from build123d import *

# Parameters (mm, degrees)
F0_R     = 4.699
F1_DEPTH = 19.05
F2_DEPTH = 50.8
F3_DEPTH = 25.4


# Not quite as in the source:
# - a feature of the source that left no trace in its solid (it failed there, or was rolled back) is left out


with BuildPart() as f1:
    # F0 (on Top) → F1 (new body)
    with BuildSketch(Plane.XY):
        Polygon((46.0592823896, 54.4316620976), (-30.1407176104, 54.4316620976), (-30.1407176104, 29.0316620976), (-6.3155176104, 29.0316620976), (22.2340823896, 29.0316620976), (46.0592823896, 29.0316620976), align=None)
        with Locations((-17.4028014716, 41.883985333)):
            Circle(F0_R, mode=Mode.SUBTRACT)
        with Locations((33.3109036978, 41.7761531395)):
            Circle(F0_R, mode=Mode.SUBTRACT)
        Polygon((-6.3155176104, 29.0316620976), (-30.1407176104, 29.0316620976), (-30.1407176104, 3.6316620976), (-6.3155176104, 3.6316620976), (-6.3155176104, 16.6544260591), align=None)
        Polygon((-6.3155176104, 3.6316620976), (-30.1407176104, 3.6316620976), (-30.1407176104, -27.9789566994), (-30.1407176104, -40.8183379024), (-23.7907176104, -40.8183379024), (-17.4407176104, -40.8183379024), (33.3592823896, -40.8183379024), (46.0592823896, -40.8183379024), (46.0592823896, -28.1183379024), (46.0592823896, 3.6316620976), (22.2340823896, 3.6316620976), align=None)
        with Locations((-17.4763201279, -28.1499404974)):
            Circle(F0_R, mode=Mode.SUBTRACT)
        with Locations((33.0586231201, -27.9913925288)):
            Circle(F0_R, mode=Mode.SUBTRACT)
        Polygon((46.0592823896, 3.6316620976), (46.0592823896, 29.0316620976), (22.2340823896, 29.0316620976), (22.2340823896, 18.1238111109), (22.2340823896, 3.6316620976), align=None)
    extrude(amount=F1_DEPTH)

    # F0 (on Top) → F2 (join)
    with BuildSketch(Plane.XY):
        Polygon((-6.3155176104, 29.0316620976), (-30.1407176104, 29.0316620976), (-30.1407176104, 3.6316620976), (-6.3155176104, 3.6316620976), (-6.3155176104, 16.6544260591), align=None)
        Polygon((46.0592823896, 3.6316620976), (46.0592823896, 29.0316620976), (22.2340823896, 29.0316620976), (22.2340823896, 18.1238111109), (22.2340823896, 3.6316620976), align=None)
    extrude(amount=F2_DEPTH)

    # F0 (on Top) → F3 (join)
    with BuildSketch(Plane.XY):
        Polygon((22.2340823896, 29.0316620976), (-6.3155176104, 29.0316620976), (-6.3155176104, 16.6544260591), (-6.3155176104, 3.6316620976), (22.2340823896, 3.6316620976), (22.2340823896, 18.1238111109), align=None)
    extrude(amount=F3_DEPTH)


solid = f1.part
For this review, take the finished solid that the model builds, in its own axes (mm). A direction names the side the tool comes from. Round coordinates to 2 decimals unless told otherwise and drop trailing zeros. Loops run counter-clockwise (first coordinate to the right, second up) from the corner with the lowest first, then second, coordinate; pieces in that order, holes last. Notation, with made-up numbers: (43, 18) - (96, 18) arc R14 cw to (96, 37) - close; hole circle Ø1 at (11.25, -15). An arc over 180 degrees is marked (long way). Use one line per item in the form item = value.
1) We need section B-B on y = 23.5. Write out the cut boundary in (x, z), then the cut area to 3 significant figures.
Solutions:
outline = (-30.14, 0) - (46.06, 0) - (46.06, 50.8) - (22.23, 50.8) - (22.23, 25.4) - (-6.32, 25.4) - (-6.32, 50.8) - (-30.14, 50.8) - close
area = 3,150 mm2
2) We need section A-A on z = 32.5. Write out the cut boundary in (x, y), then the cut area to 3 significant figures.
Solutions:
outline = (-30.14, 3.63) - (-6.32, 3.63) - (-6.32, 29.03) - (-30.14, 29.03) - close; (22.23, 3.63) - (46.06, 3.63) - (46.06, 29.03) - (22.23, 29.03) - close
area = 1,210 mm2
3) Clearance check with flat-ended pins moving along their axes: P1, Ø7.5, axis at x = 6.5, y = 22.5, coming from the +Z side; P2, Ø7.5, axis at x = 33.06, y = -27.99, coming from the -Z side; P3, Ø6, axis at x = 4.5, z = 20, coming from the -Y side; P4, Ø12, axis at x = 11, z = 31, coming from the +Y side. State where each tip first meets the part, or that it passes through.
Solutions:
P1 = 25.4
P2 = through
P3 = -40.82
P4 = 29.03
4) Wall thickness on probe 1 along X at (y, z) = (7, 32.5); probe 2 along Y at (x, z) = (-15, 5); probe 3 along Y at (x, z) = (-18, 18.5): over which ranges is each line inside the solid? List them lowest first.
Solutions:
probe_1 = -30.14 to -6.32, 22.23 to 46.06
probe_2 = -40.82 to -32.14, -24.16 to 37.85, 45.92 to 54.43
probe_3 = -40.82 to -32.82, -23.48 to 37.22, 46.54 to 54.43
5) Mouldability with a two-part tool opening along X and no side actions: class faces 1 (the face through (7, 42, 19.05)), 2 (the face through (22.234, 17, 38)), 3 (the face through (-30.141, 7, 19)) as pulls with the +X half, pulls with the -X half, needs draft (parallel to the pull), parting line crosses it, or undercut.
Solutions:
face_1 = needs draft
face_2 = undercut
face_3 = pulls with the -X half
6) We need section C-C on x = 12.5. Write out the cut boundary in (y, z).
Solutions:
outline = (-40.82, 0) - (54.43, 0) - (54.43, 19.05) - (29.03, 19.05) - (29.03, 25.4) - (3.63, 25.4) - (3.63, 19.05) - (-40.82, 19.05) - close
7) We need section D-D on z = 11.5. Write out the cut boundary in (x, y).
Solutions:
outline = (-30.14, -40.82) - (46.06, -40.82) - (46.06, 54.43) - (-30.14, 54.43) - close; hole circle Ø9.4 at (-17.48, -28.15); hole circle Ø9.4 at (-17.4, 41.88); hole circle Ø9.4 at (33.06, -27.99); hole circle Ø9.4 at (33.31, 41.78)
8) Tool access review of faces 4 (the face through (7, 3.632, 24)), 5 (the face through (-6.316, 16, 38)), 6 (the face through (8, 29.032, 24)): name each direction out of +Z, -Z, +X, -X, +Y, -Y from which nothing blocks a thin tool from reaching the whole face with its end or side.
Solutions:
face_4 = +Z, +X, -X, -Y
face_5 = +Z, +Y, -Y
face_6 = +Z, +X, -X, +Y
